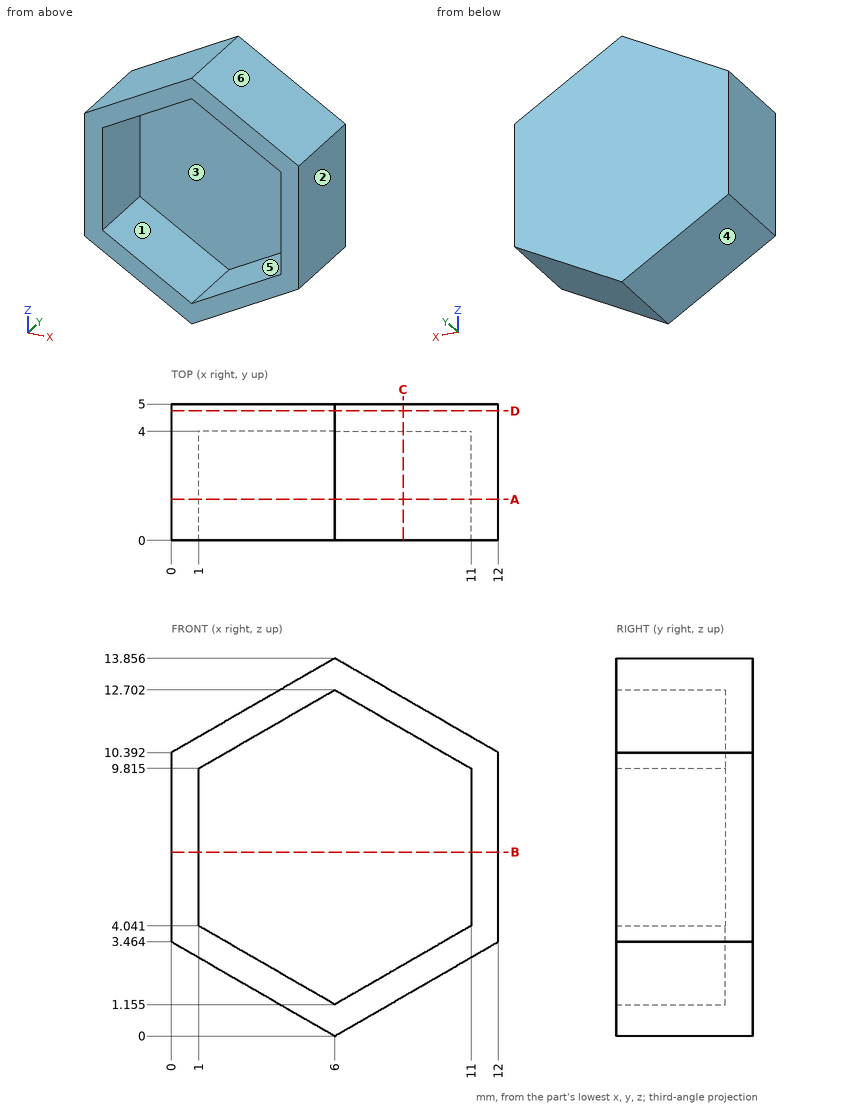
Part print with two shaded views. Sizes in mm from the minimum x, y, z corner. A direction names the side the tool comes from. Coordinates: 2 decimals unless noted, no trailing zeros. Order: outer loops, then holes, each group sorted by start corner. A loop starts at its lowest first (then second) coordinate and runs counter-clockwise, first axis right, second up. Notation, with made-up numbers: M -11,-12 L 42,-12 A12 ccw 42,8 Z; hole C 38.5,77.25 d7. An arc over 180 degrees is marked long. One line per question, with ' | ' between items. Start each with the question number.
1. Cut at A-A (y = 1.5). Write the cut outline in (x, z) (1 decimal).
2. Cut at D-D (y = 4.75). Write the cut outline in (x, z) (1 decimal).
3. Tool access for the marked faces 1 and 2: list every direction of +Z, -Z, +X, -X, +Y, -Y with a clear straight run to the whole face (end or side of a thin tool).
4. Cut at C-C (x = 8.5). Write the cut outline in (y, z).
5. Mould opens along Z. For the marked faces 3, 4, 5 and 6 say: +Z half, -Z half, draft (parallel to the pull), parting line (faces both ways), or undercut.
6. Wall check: line 1 along X through (y, z) = (2.05, 5); line 2 along Y through (x, z) = (8.5, 4); line 3 along Z through (x, y) = (7.5, 1.9) (1 decimal). Give the ranges that are in metal, low to high. Write a range as [from, to].
7. Flat gauge pin, fed straight in: P1, Ø1, axis at x = 9.5, z = 6, coming from the -Y side. Where does the tip first touch, or does it go through?
8. Cut at B-B (z = 6.75). Write the cut outline in (x, y), plus the area to 3 significant figures.
The answers:
1) outline: M 0,3.5 L 6,0 L 12,3.5 L 12,10.4 L 6,13.9 L 0,10.4 Z; hole M 1,4 L 6,1.2 L 11,4 L 11,9.8 L 6,12.7 L 1,9.8 Z
2) outline: M 0,3.5 L 6,0 L 12,3.5 L 12,10.4 L 6,13.9 L 0,10.4 Z
3) face 1: -Y | face 2: +Z, -Z, +X, +Y, -Y
4) outline: M 0,1.44 L 5,1.44 L 5,12.41 L 0,12.41 L 0,11.26 L 4,11.26 L 4,2.6 L 0,2.6 Z
5) face 3: undercut | face 4: -Z half | face 5: undercut | face 6: +Z half
6) line 1: x = [0, 1], [11, 12] | line 2: y = [4, 5] | line 3: z = [0.9, 2], [11.8, 13]
7) P1: stops at y = 4
8) outline: M 0,0 L 1,0 L 1,4 L 11,4 L 11,0 L 12,0 L 12,5 L 0,5 Z | area: 20.0 mm2
